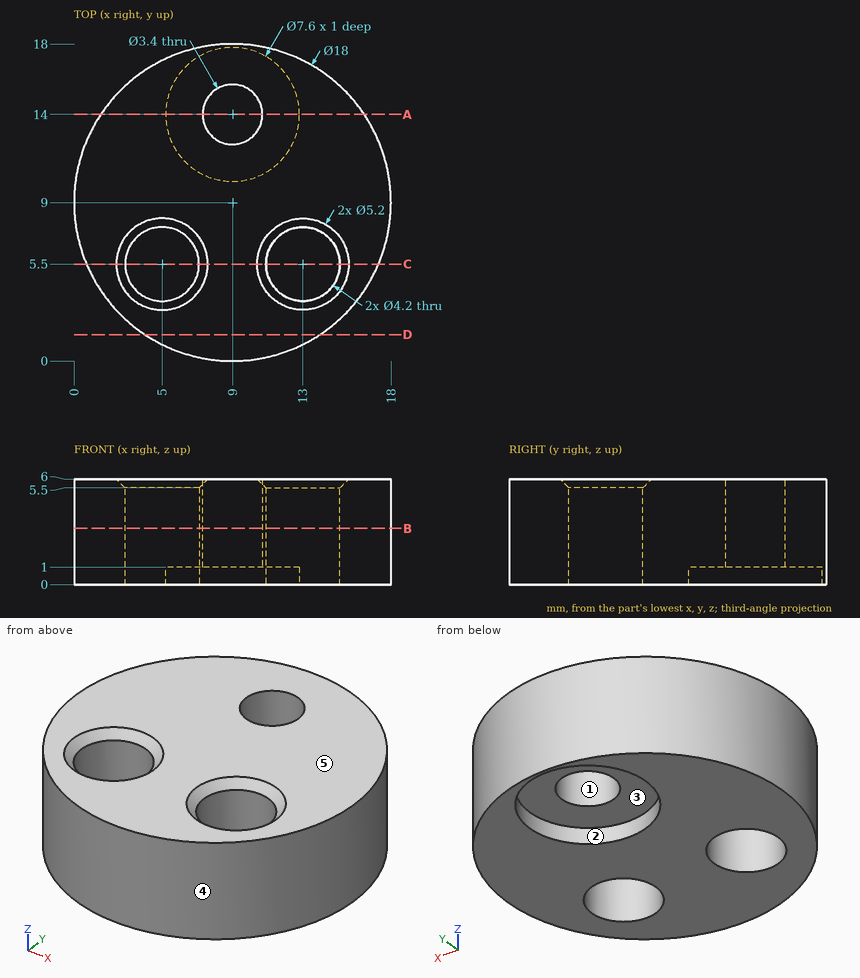
Input: dimensioned drawing with shaded views. Units: mm. Origin: part minimum x, y, z. A direction names the side the tool comes from. Round coordinates to 2 decimals unless told otherwise and drop trailing zeros. Loops run counter-clockwise (first coordinate to the right, second up) from the corner with the lowest first, then second, coordinate; pieces in that order, holes last. Notation, with made-up numbers: (86.5, 31.25) -> (97.5, 31.25) arc R15 cw to (97.5, 42.25) -> close; hole circle Ø7 at (-32.5, 43). An arc over 180 degrees is marked (long way). Answer as a JSON object with one key per item and string values. Group by question number.
1) Ray query, L1, parallel to Y at x = 9, z = 0.4; L2, parallel to X at y = 4.25, z = 4; L3, parallel to Y at x = 5.5, z = 3.75. Return the intervals inside material, ascending.
2) Reachability of the marked faces 1 and 2 from +Z, -Z, +X, -X, +Y, -Y: full face, straight path, thin tool, end or side. Return the list, or none.
3) Section query B-B on z = 3.2. Output: boundary loops of the cut face in (x, y).
4) Section query D-D on y = 1.5. Output: boundary loops of the cut face in (x, z), plus the area to 3 significant figures.
5) Section query A-A on y = 14. Output: boundary loops of the cut face in (x, z).
6) Pin query (flat end, axial travel): pin 1 (1.5 mm diameter, centred on y = 14.5, z = 4, fed in from +X); pin 2 (1 mm diameter, centred on x = 10, y = 13.5, fed in from +Z); pin 3 (6 mm diameter, centred on x = 9, y = 14, fed in from -Z). Return the tip coordinate at first contact, or that it passes through.
7) Section query C-C on y = 5.5. Output: boundary loops of the cut face in (x, z).
8) Draft query along Y for the marked faces 3, 4 and 5. Return one class per face: +Y half, -Y half, draft (parallel to the pull), parting line (faces both ways), or undercut.
Reply:
{
 "1": {"L1": "y = 0 to 10.2, 17.8 to 18", "L2": "x = 1.36 to 3.31, 6.69 to 11.31, 14.69 to 16.64", "L3": "y = 0.71 to 3.46, 7.54 to 17.29"},
 "2": {"face 1": "+Z, -Z", "face 2": "-Z"},
 "3": {"outline": "circle Ø18 at (9, 9); hole circle Ø4.2 at (5, 5.5); hole circle Ø3.4 at (9, 14); hole circle Ø4.2 at (13, 5.5)"},
 "4": {"outline": "(4.03, 0) -> (13.97, 0) -> (13.97, 6) -> (4.03, 6) -> close", "area": "59.7 mm2"},
 "5": {"outline": "(1.52, 0) -> (5.2, 0) -> (5.2, 1) -> (7.3, 1) -> (7.3, 6) -> (1.52, 6) -> close; (10.7, 1) -> (12.8, 1) -> (12.8, 0) -> (16.48, 0) -> (16.48, 6) -> (10.7, 6) -> close"},
 "6": {"pin 1": "stops at x = 16.64", "pin 2": "passes through", "pin 3": "stops at z = 1"},
 "7": {"outline": "(0.71, 0) -> (2.9, 0) -> (2.9, 5.5) -> (2.4, 6) -> (0.71, 6) -> close; (7.1, 0) -> (10.9, 0) -> (10.9, 5.5) -> (10.4, 6) -> (7.6, 6) -> (7.1, 5.5) -> close; (15.1, 0) -> (17.29, 0) -> (17.29, 6) -> (15.6, 6) -> (15.1, 5.5) -> close"},
 "8": {"face 3": "undercut", "face 4": "parting line", "face 5": "draft"}
}
